Model file for the job. Use its own axes, mm. Face numbers are marked on the shaded views. Give positions to 0.01 mm unless a question says otherwise; leave off trailing zeros. Order: outer loops, then holes, each group sorted by start corner. A loop starts at its lowest first (then second) coordinate and runs counter-clockwise, first axis right, second up. Notation, with made-up numbers: (-35.75, -11) -> (-6.75, -11) arc R12 cw to (-6.75, -3) -> close; hole circle Ø8 at (59, 63). An arc over 180 degrees is marked (long way). Use CSV: the item, a comma, the result in double quotes. Start each with the question number.
1. Pull direction Z, two halves, no side cores. Call the marked faces 1, 2 and 3: released by +Z, released by -Z, zero draft, split by the parting line, or undercut.
2. Wall check: line 1 (Y direction, x = 4, z = 0.25); line 2 (Y direction, x = 1.5, z = -1.25) (3 decimals); line 3 (Y direction, x = 2.25, z = 0.75) (3 decimals). Give the ranges that are in metal, low to high. Write a range as from..to.
3. Drop flat-ended pins along their axis: pin 1 (3 mm diameter, centred on x = 8.5, y = -0.5, fed in from +Z); pin 2 (4 mm diameter, centred on x = 9, z = -1, fed in from -Y); pin 3 (3 mm diameter, centred on x = 1.5, y = 2.5, fed in from +Z). Give the stop position or say it passes through.
4. Cut at A-A on x = 7. List the corners of the cut face in (y, z).
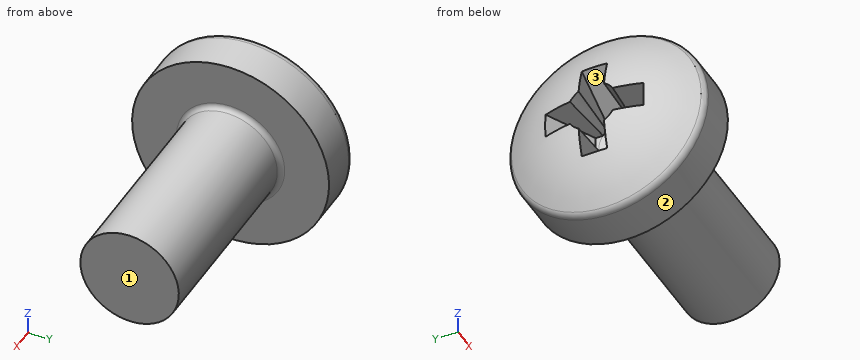
```python
from build123d import *

# Parameters (mm, degrees)
FILLET1_R    = 0.2
SKETCH3_W    = 1.03
SKETCH3_H    = 4.3
SKETCH4_W    = 1.03
SKETCH4_H    = 1.966638154
RECPAT_COUNT = 2
RECPAT_ANGLE = 90


with BuildPart() as part:
    # BodySke → Base-Revolve (revolve)
    with BuildSketch(Plane.XY, mode=Mode.PRIVATE) as base_revolve_sk:
        with BuildLine():
            Line((3.1, 2), (3.1, 4))
            Line((3.1, 4), (1.555305874, 4))
            ThreePointArc((1.555305874, 4), (1.392873227, 3.961271902), (1.265388955, 3.853420195))
            ThreePointArc((1.265388955, 3.853420195), (0.324444487, 2.027933456), (0, 0))
            Line((0, 0), (11.1, 0))
            Line((11.1, 0), (11.1, 2))
            Line((11.1, 2), (3.1, 2))
        make_face()
    revolve(base_revolve_sk.sketch.rotate(Axis((-25.4, 0, 0), (1, 0, 0)), 90), axis=Axis((-25.4, 0, 0), (1, 0, 0)))  # turned: the seam where the file's is

    # Fillet1
    fillet1_edges = [part.edges().sort_by_distance(p)[0] for p in [
        (3.1, 0, -2),
    ]]
    fillet(fillet1_edges, radius=FILLET1_R)

    # Sketch3 → Recess section 0
    with BuildSketch(Plane(origin=(0, 0, 0), x_dir=(0, 0, -1), z_dir=(1, 0, 0))):
        Rectangle(SKETCH3_W, SKETCH3_H)
    # Sketch4 → Recess section 1
    with BuildSketch(Plane(origin=(2.34, 0, 0), x_dir=(0, 0, -1), z_dir=(1, 0, 0))):
        Rectangle(SKETCH4_W, SKETCH4_H)
    recess = loft(mode=Mode.SUBTRACT)

    # RecPat: Recess ×2 about axis
    recpat_axis = Axis((-25.4, 0, 0), (1, 0, 0))
    for i in range(1, RECPAT_COUNT):
        add(recess.rotate(recpat_axis, i * RECPAT_ANGLE / (RECPAT_COUNT - 1)), mode=Mode.SUBTRACT)

    # RecCorSke → RecessCore (revolve, cut)
    with BuildSketch(Plane.XY, mode=Mode.PRIVATE) as recesscore_sk:
        Polygon((0, 0), (0, 1.01462874), (2.34, 0.851), (2.616506661, 0), align=None)
    revolve(recesscore_sk.sketch.rotate(Axis((-3.175, 0, 0), (1, 0, 0)), 90), axis=Axis((-3.175, 0, 0), (1, 0, 0)), mode=Mode.SUBTRACT)  # turned: the seam where the file's is


solid = part.part
```
Verdict:
1,face 1,"zero draft"
1,face 2,"split by the parting line"
1,face 3,"undercut"
2,line 1,"-1.98..1.98"
2,line 2,"-3.795..-0.515, 0.515..3.795"
2,line 3,"-3.929..-0.515, 0.515..3.929"
3,pin 1,"z = 2"
3,pin 2,"y = -2"
3,pin 3,"z = 3.87"
4,outline,"circle Ø4 at (0, 0)"
